Geometry: final body of the model. Coordinates: model frame, mm. A direction names the side the tool comes from. Round coordinates to 2 decimals unless told otherwise and drop trailing zeros. Loops run counter-clockwise (first coordinate to the right, second up) from the corner with the lowest first, then second, coordinate; pieces in that order, holes last. Notation, with made-up numbers: (15.25, -4.5) - (62.25, -4.5) arc R23 ccw to (62.25, 14.5) - close; hole circle Ø7 at (78, -3). An arc over 180 degrees is marked (long way). Use CSV: the item, a comma, the result in double quotes.
from build123d import *

# Parameters (mm, degrees)
BOSS_EXTRUDE1_DEPTH = 55
SHELL1_START        = 3
SHELL1_DEPTH        = 49


# Read off the part's stored shape, not the designer's step: Shell1
with BuildPart() as part:
    # Sketch2 → Boss-Extrude1 (new body)
    with BuildSketch(Plane(origin=(0, 0, 0), x_dir=(1, 0, 0), z_dir=(0, 1, 0))):
        Polygon((9, 55), (0, 46), (0, 9), (9, 0), (85, 0), (140, 0), (140, 46), (131, 55), align=None)
        Polygon((140, 0), (85, 0), (85, -46), (94, -55), (131, -55), (140, -46), align=None)
    extrude(amount=BOSS_EXTRUDE1_DEPTH)

    # Shell1 outline → Shell1 (cut)
    with BuildSketch(Plane(origin=(0, 0, 0), x_dir=(1, 0, 0), z_dir=(0, 1, 0)).offset(SHELL1_START)):
        Polygon((10.242640687, 3), (88, 3), (88, -44.757359313), (95.242640687, -52), (129.757359313, -52), (137, -44.757359313), (137, 44.757359313), (129.757359313, 52), (10.242640687, 52), (3, 44.757359313), (3, 10.242640687), align=None)
    extrude(amount=SHELL1_DEPTH, mode=Mode.SUBTRACT)


solid = part.part
Item 1: Section C-C on z = -28.5. Return the cut outline in (x, y).
Final values:
outline,"(0, 0) - (140, 0) - (140, 55) - (0, 55) - close; hole (3, 3) - (137, 3) - (137, 52) - (3, 52) - close"
Item 2: Section B-B on y = 44. Return the cut outline in (x, z), plus the area to 3 significant figures.
Final values:
outline,"(0, -46) - (9, -55) - (131, -55) - (140, -46) - (140, 46) - (131, 55) - (94, 55) - (85, 46) - (85, 0) - (9, 0) - (0, -9) - close; hole (3, -44.76) - (10.24, -52) - (129.76, -52) - (137, -44.76) - (137, 44.76) - (129.76, 52) - (95.24, 52) - (88, 44.76) - (88, -3) - (10.24, -3) - (3, -10.24) - close"
area,"1,390 mm²"
Item 3: Section A-A on x = 123. Return the cut outline in (y, z), plus the area to 3 significant figures.
Final values:
outline,"(0, -55) - (55, -55) - (55, 55) - (0, 55) - close; hole (3, -52) - (52, -52) - (52, 52) - (3, 52) - close"
area,"954 mm²"
Item 4: Material intervals for line 1 (Y direction, x = 123, z = -15.5); line 2 (Z direction, x = 34.5, y = 8); line 3 (X direction, y = 47.5, z = 34.5), sorted ascending.
Final values:
line 1,"y = 0 to 3, 52 to 55"
line 2,"z = -55 to -52, -3 to 0"
line 3,"x = 85 to 88, 137 to 140"
Item 5: Reachability of faces 1 (the flat face through (135, 27, 51)), 2 (the flat face through (85, 27, 23)), 3 (the flat face through (6.57, 27.16, -6.67)) from +Z, -Z, +X, -X, +Y, -Y: full face, straight path, thin tool, end or side. Return the list, or none.
Final values:
face 1,"+Z, +X, +Y, -Y"
face 2,"+Z, -X, +Y, -Y"
face 3,"none"
Item 6: Mould query, pull axis Z, two halves, no side actions, for faces 4 (the flat face through (89, 27, 50)), 5 (the flat face through (91.57, 27.16, 48.33)), 6 (the flat face through (140, 27, 1)), 7 (the flat face through (136, 27, -50)). Classes: released by +Z, released by -Z, zero draft, split by the parting line, or undercut.
Final values:
face 4,"released by +Z"
face 5,"undercut"
face 6,"zero draft"
face 7,"released by -Z"
Item 7: Pin query (flat end, axial travel): P1, Ø24.5, axis at x = 71, y = 39.5, coming from the +Z side; P2, Ø23, axis at y = 41, z = 24.5, coming from the -X side. Return the tip coordinate at first contact, or that it passes through.
Final values:
P1,"stops at z = 0"
P2,"stops at x = 85"
